Check sheet for the modelled part. Datum: model origin and axes. Units: mm. A direction names the side the tool comes from. Give positions to 0.01 mm unless a question says otherwise; leave off trailing zeros. Order: outer loops, then holes, each group sorted by start corner. A loop starts at its lowest first (then second) coordinate and runs counter-clockwise, first axis right, second up.
```python
from build123d import *

# Parameters (mm, degrees)
BOSS_EXTRUDE1_DEPTH            = 6
SKETCH3_R                      = 1.75
CUT_EXTRUDE2_DEPTH             = 69.176242196
BOSS_EXTRUDE2_DEPTH            = 13
BOSS_EXTRUDE3_DEPTH            = 6
CUT_EXTRUDE3_REACH             = 74.367
SKETCH6_R                      = 1.75
CUT_EXTRUDE4_REACH             = 74.367
SKETCH8_R                      = 15.1
BOSS_EXTRUDE4_DEPTH            = 11
SKETCH9_R                      = 1.75
CUT_EXTRUDE5_DEPTH             = 10
CUT_EXTRUDE6_REACH             = 78.864
SKETCH11_R                     = 3
CUT_EXTRUDE6_DIRECTION_2_DEPTH = 77.863515556
CUT_EXTRUDE7_REACH             = 74.719
SKETCH12_R                     = 3


with BuildPart() as part:
    # Sketch1 → Boss-Extrude1 (new body)
    with BuildSketch(Plane(origin=(0, 0, 0), x_dir=(1, 0, 0), z_dir=(0, 1, 0))):
        with BuildLine():
            Line((-50, 16), (50, 16))
            ThreePointArc((50, 16), (66, 0), (50, -16))
            Line((50, -16), (-50, -16))
            ThreePointArc((-50, -16), (-66, 0), (-50, 16))
        make_face()
    extrude(amount=BOSS_EXTRUDE1_DEPTH)

    # Sketch3 → Cut-Extrude2 (cut, through all)
    with BuildSketch(Plane.XZ):
        with Locations(Location((50, 0, 0), (0, 0, 270))):
            Circle(SKETCH3_R)
    extrude(amount=-CUT_EXTRUDE2_DEPTH, mode=Mode.SUBTRACT)

    # Sketch4 → Boss-Extrude2 (add)
    with BuildSketch(Plane(origin=(0, 6, 0), x_dir=(1, 0, 0), z_dir=(0, 1, 0))):
        with BuildLine():
            Line((-50, 16), (15, 16))
            Line((15, 16), (15, -16))
            Line((15, -16), (-50, -16))
            ThreePointArc((-50, -16), (-66, 0), (-50, 16))
        make_face()
    extrude(amount=BOSS_EXTRUDE2_DEPTH)

    # Sketch5 → Boss-Extrude3 (add)
    with BuildSketch(Plane(origin=(0, 19, 0), x_dir=(1, 0, 0), z_dir=(0, 1, 0))):
        with BuildLine():
            Line((-50, 16), (50, 16))
            ThreePointArc((50, 16), (66, 0), (50, -16))
            Line((50, -16), (-50, -16))
            ThreePointArc((-50, -16), (-66, 0), (-50, 16))
        make_face()
    extrude(amount=BOSS_EXTRUDE3_DEPTH)

    # Sketch6 → Cut-Extrude3 (cut, up to next)
    with BuildSketch(Plane(origin=(0, 25, 0), x_dir=(1, 0, 0), z_dir=(0, 1, 0)), mode=Mode.PRIVATE) as cut_extrude3_sk1:
        with Locations(Location((50, 0, 0), (0, 0, 90))):
            Circle(SKETCH6_R)
    cut_extrude3_tool1 = extrude(cut_extrude3_sk1.sketch, amount=-CUT_EXTRUDE3_REACH, mode=Mode.PRIVATE) & part.part
    add(cut_extrude3_tool1.solids().sort_by_distance((50, 25, 0))[0], mode=Mode.SUBTRACT)

    # Sketch7 → Cut-Extrude4 (cut, up to next)
    with BuildSketch(Plane(origin=(0, 25, 0), x_dir=(1, 0, 0), z_dir=(0, 1, 0)), mode=Mode.PRIVATE) as cut_extrude4_sk1:
        with BuildLine():
            ThreePointArc((-37.731263809, -10.270253759), (-43.22962557, -14.496966237), (-50, -16))
            Line((-50, -16), (50, -16))
            add(Edge.make_bspline(
                [(-37.731263809, -10.270253759), (-30.332556703, -1.431836739), (6.050402888, -3.364587973), (38.512231583, -16), (50, -16)],
                knots=[0, 0, 0, 0, 0.426660683, 1, 1, 1, 1], degree=3))
        make_face()
    cut_extrude4_tool1 = extrude(cut_extrude4_sk1.sketch, amount=-CUT_EXTRUDE4_REACH, mode=Mode.PRIVATE) & part.part
    add(cut_extrude4_tool1.solids().sort_by_distance((-6.915299, 25, 11.013102))[0], mode=Mode.SUBTRACT)

    # Sketch8 → Boss-Extrude4 (add)
    with BuildSketch(Plane.XZ):
        with Locations(Location((-50, 0, 0), (0, 0, 90))):
            Circle(SKETCH8_R)
    extrude(amount=BOSS_EXTRUDE4_DEPTH)

    # Sketch9 → Cut-Extrude5 (cut)
    with BuildSketch(Plane.XZ.offset(11)):
        with Locations(Location((-50, 6.75, 0), (0, 0, 270))):
            Circle(SKETCH9_R)
        with Locations(Location((-50, -6.75, 0), (0, 0, 270))):
            Circle(SKETCH9_R)
    extrude(amount=-CUT_EXTRUDE5_DEPTH, mode=Mode.SUBTRACT)

    # Sketch11 → Cut-Extrude6 (cut, up to next)
    with BuildSketch(Plane.XZ.offset(11), mode=Mode.PRIVATE) as cut_extrude6_sk1:
        with Locations(Location((-50, 0, 0), (0, 0, 90))):
            Circle(SKETCH11_R)
    cut_extrude6_tool1 = extrude(cut_extrude6_sk1.sketch, amount=-CUT_EXTRUDE6_REACH, mode=Mode.PRIVATE) & part.part
    add(cut_extrude6_tool1.solids().sort_by_distance((-50, -11, 0))[0], mode=Mode.SUBTRACT)

    # Sketch11 → Cut-Extrude6 direction 2 (cut)
    with BuildSketch(Plane.XZ.offset(11)):
        with Locations(Location((-50, 0, 0), (0, 0, 90))):
            Circle(SKETCH11_R)
    extrude(amount=CUT_EXTRUDE6_DIRECTION_2_DEPTH, mode=Mode.SUBTRACT)

    # Sketch12 → Cut-Extrude7 (cut, up to next)
    with BuildSketch(Plane.XZ.offset(1), mode=Mode.PRIVATE) as cut_extrude7_sk1:
        with Locations(Location((-50, 6.75, 0), (0, 0, 270))):
            Circle(SKETCH12_R)
    cut_extrude7_tool1 = extrude(cut_extrude7_sk1.sketch, amount=-CUT_EXTRUDE7_REACH, mode=Mode.PRIVATE) & part.part
    # Sketch12 → Cut-Extrude7 (cut, up to next)
    with BuildSketch(Plane.XZ.offset(1), mode=Mode.PRIVATE) as cut_extrude7_sk2:
        with Locations(Location((-50, -6.75, 0), (0, 0, 270))):
            Circle(SKETCH12_R)
    cut_extrude7_tool2 = extrude(cut_extrude7_sk2.sketch, amount=-CUT_EXTRUDE7_REACH, mode=Mode.PRIVATE) & part.part
    add(cut_extrude7_tool1.solids().sort_by_distance((-50, -1, 6.75))[0], mode=Mode.SUBTRACT)
    add(cut_extrude7_tool2.solids().sort_by_distance((-50, -1, -6.75))[0], mode=Mode.SUBTRACT)


solid = part.part
```
Q1. Sectioned sample at D-D, the plane y = 4.5. Count the separate pieces of the cut face and the enclosed holes in it, plus the area to 3 significant figures.
Q2. Sectioned sample at C-C, the plane y = -4.5. Record the cut outline in (x, z), plus the area to 3 significant figures.
Q3. Go/stop test with flat-tipped pins: P1, Ø1, axis at y = 4, z = 6.5, coming from the +X side; P2, Ø4, axis at x = -50, z = -6.75, coming from the +Y side; P3, Ø10.5, axis at y = 13, z = -5, coming from the +X side. Record where each tip stops, or that it passes through.
Q4. Material ranges on line 1 (X direction, y = 4, z = 0); line 2 (Y direction, x = 48, z = 11); line 3 (X direction, y = -3.75, z = 6.75), recorded low to high.
Q5. Sectioned sample at B-B, the plane z = -6.75. Record the cut outline in (x, y).
Q6. Tool access check on faces 1 (the flat face through (-52, -1, -7)), 2 (the flat face through (41, 19, 0)), 3 (the cylindrical face through (-64.97, -5.42, -1.97)), 4 (the cylindrical face through (48.29, 2.96, 0.38)). Record the directions out of +Z, -Z, +X, -X, +Y, -Y that give a thin tool (end or side, any length) a straight path to the whole face; none if there is none.
Q7. Draft check along Y on faces 5 (the flat face through (16, 0, -4)), 6 (the cylindrical face through (-51.71, -6.07, 7.13)), 7 (the flat face through (41, 6, 0)), 8 (the flat face through (1, 25, -4)). Enter one of: pulls with the +Y half, pulls with the -Y half, needs draft (parallel to the pull), parting line crosses it, or undercut.
Q8. Sectioned sample at A-A, the plane z = 0. Record the cut outline in (x, y), plus the area to 3 significant figures.
Filled in:
1. separate pieces: 1
1. enclosed holes: 4
1. area: 3,200 mm2
2. outline: circle Ø30.2 at (-50, 0); hole circle Ø6 at (-50, 0); hole circle Ø3.5 at (-50, -6.75); hole circle Ø3.5 at (-50, 6.75)
2. area: 669 mm2
3. P1: stops at x = 64.83
3. P2: stops at y = -1
3. P3: stops at x = 15
4. line 1: x = -66 to -53, -47 to 48.25, 51.75 to 66
4. line 2: y = 0 to 6, 19 to 25
4. line 3: x = -63.51 to -51.75, -48.25 to -36.49
5. outline: (-64.51, 0) - (-63.51, 0) - (-63.51, -11) - (-51.75, -11) - (-51.75, -1) - (-53, -1) - (-53, 25) - (-64.51, 25) - close; (-48.25, -11) - (-36.49, -11) - (-36.49, 0) - (64.51, 0) - (64.51, 6) - (15, 6) - (15, 19) - (64.51, 19) - (64.51, 25) - (-47, 25) - (-47, -1) - (-48.25, -1) - close
6. face 1: +Y
6. face 2: +Z, -Z, +X
6. face 3: -Y
6. face 4: +Y, -Y
7. face 5: pulls with the -Y half
7. face 6: needs draft
7. face 7: undercut
7. face 8: pulls with the +Y half
8. outline: (-66, 0) - (-65.1, 0) - (-65.1, -11) - (-53, -11) - (-53, 25) - (-66, 25) - close; (-47, -11) - (-34.9, -11) - (-34.9, 0) - (48.25, 0) - (48.25, 6) - (15, 6) - (15, 19) - (48.25, 19) - (48.25, 25) - (-47, 25) - close; (51.75, 0) - (66, 0) - (66, 6) - (51.75, 6) - close; (51.75, 19) - (66, 19) - (66, 25) - (51.75, 25) - close
8. area: 2,710 mm2
